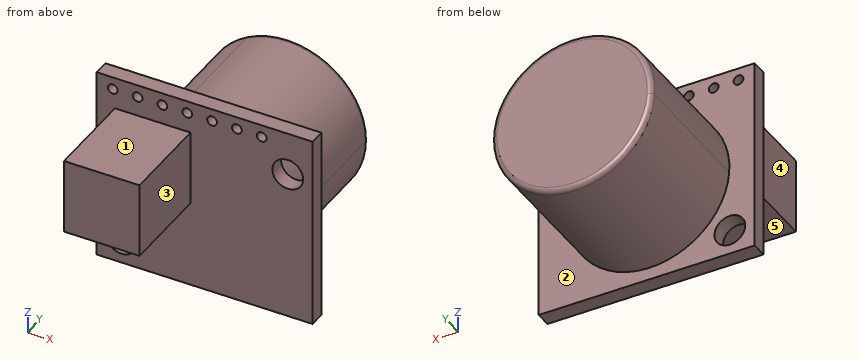
```python
from build123d import *

# Parameters (mm, degrees)
SKETCH1_W           = 22.098
SKETCH1_H           = 19.939
SKETCH1_R           = 0.5
SKETCH1_R_2         = 1.5748
BOSS_EXTRUDE1_DEPTH = 1.6002
SKETCH1_3_W         = 7.7216
SKETCH1_3_H         = 7.7216
BOSS_EXTRUDE2_DEPTH = 9.3472
BOSS_EXTRUDE3_DEPTH = 15.7734
FILLET1_R           = 0.5


with BuildPart() as part:
    # Sketch1 → Boss-Extrude1 (new body)
    # profile 1 of 6: a face of its own
    with BuildSketch(Plane(origin=(0, 0, 0), x_dir=(1, 0, 0), z_dir=(0, 1, 0))):
        with Locations((11.049, 9.9695)):
            Rectangle(SKETCH1_W, SKETCH1_H)
        with Locations(Location((1.651, 1.27, 0), (0, 0, 270))):
            Circle(SKETCH1_R, mode=Mode.SUBTRACT)
        with Locations(Location((4.191, 1.27, 0), (0, 0, 270))):
            Circle(SKETCH1_R, mode=Mode.SUBTRACT)
        with Locations(Location((6.731, 1.27, 0), (0, 0, 270))):
            Circle(SKETCH1_R, mode=Mode.SUBTRACT)
        with Locations(Location((9.271, 1.27, 0), (0, 0, 270))):
            Circle(SKETCH1_R, mode=Mode.SUBTRACT)
        with Locations(Location((11.811, 1.27, 0), (0, 0, 270))):
            Circle(SKETCH1_R, mode=Mode.SUBTRACT)
        with Locations(Location((14.351, 1.27, 0), (0, 0, 270))):
            Circle(SKETCH1_R, mode=Mode.SUBTRACT)
        with Locations(Location((16.891, 1.27, 0), (0, 0, 270))):
            Circle(SKETCH1_R, mode=Mode.SUBTRACT)
        with Locations(Location((19.558, 4.445, 0), (0, 0, 270))):
            Circle(SKETCH1_R_2, mode=Mode.SUBTRACT)
        with BuildLine():
            Line((1.8796, 3.302), (1.8796, 11.0236))
            Line((1.8796, 11.0236), (2.600005352, 11.0236))
            ThreePointArc((2.600005352, 11.0236), (11.040962011, 18.677352606), (18.965620393, 10.4902))
            ThreePointArc((18.965620393, 10.4902), (14.952824562, 3.444697625), (6.845958862, 3.302))
            Line((6.845958862, 3.302), (1.8796, 3.302))
        make_face(mode=Mode.SUBTRACT)
        with Locations(Location((2.54, 17.399, 0), (0, 0, 270))):
            Circle(SKETCH1_R_2, mode=Mode.SUBTRACT)
    # profile 2 of 6: a face of its own
    with BuildSketch(Plane(origin=(0, 0, 0), x_dir=(1, 0, 0), z_dir=(0, 1, 0))):
        with BuildLine():
            Line((2.600005352, 11.0236), (1.8796, 11.0236))
            Line((1.8796, 11.0236), (1.8796, 3.302))
            Line((1.8796, 3.302), (6.845958862, 3.302))
            ThreePointArc((6.845958862, 3.302), (3.596234131, 6.543223808), (2.600005352, 11.0236))
        make_face()
    # profile 3 of 6: a face of its own
    with BuildSketch(Plane(origin=(0, 0, 0), x_dir=(1, 0, 0), z_dir=(0, 1, 0))):
        with BuildLine():
            ThreePointArc((18.965620393, 10.4902), (11.040962011, 18.677352606), (2.600005352, 11.0236))
            Line((2.600005352, 11.0236), (9.6012, 11.0236))
            Line((9.6012, 11.0236), (9.6012, 3.302))
            Line((9.6012, 3.302), (6.845958862, 3.302))
            ThreePointArc((6.845958862, 3.302), (14.952824562, 3.444697625), (18.965620393, 10.4902))
        make_face()
    # profile 4 of 6: a face of its own
    with BuildSketch(Plane(origin=(0, 0, 0), x_dir=(1, 0, 0), z_dir=(0, 1, 0))):
        with BuildLine():
            Line((9.6012, 11.0236), (2.600005352, 11.0236))
            ThreePointArc((2.600005352, 11.0236), (3.596234131, 6.543223808), (6.845958862, 3.302))
            Line((6.845958862, 3.302), (9.6012, 3.302))
            Line((9.6012, 3.302), (9.6012, 11.0236))
        make_face()
    # profile 5 of 6: a face of its own
    with BuildSketch(Plane(origin=(0, 0, 0), x_dir=(1, 0, 0), z_dir=(0, 1, 0))):
        with BuildLine():
            ThreePointArc((18.965620393, 10.4902), (11.040962011, 18.677352606), (2.600005352, 11.0236))
            Line((2.600005352, 11.0236), (9.6012, 11.0236))
            Line((9.6012, 11.0236), (9.6012, 3.302))
            Line((9.6012, 3.302), (6.845958862, 3.302))
            ThreePointArc((6.845958862, 3.302), (14.952824562, 3.444697625), (18.965620393, 10.4902))
        make_face()
    # profile 6 of 6: a face of its own
    with BuildSketch(Plane(origin=(0, 0, 0), x_dir=(1, 0, 0), z_dir=(0, 1, 0))):
        with BuildLine():
            Line((9.6012, 11.0236), (2.600005352, 11.0236))
            ThreePointArc((2.600005352, 11.0236), (3.596234131, 6.543223808), (6.845958862, 3.302))
            Line((6.845958862, 3.302), (9.6012, 3.302))
            Line((9.6012, 3.302), (9.6012, 11.0236))
        make_face()
    extrude(amount=BOSS_EXTRUDE1_DEPTH)

    # Sketch1_3 → Boss-Extrude2 (add)
    with BuildSketch(Plane(origin=(0, 0, 0), x_dir=(1, 0, 0), z_dir=(0, 1, 0))):
        with Locations((5.7404, 7.1628)):
            Rectangle(SKETCH1_3_W, SKETCH1_3_H)
    extrude(amount=-BOSS_EXTRUDE2_DEPTH)

    # Sketch1_4 → Boss-Extrude3 (add)
    with BuildSketch(Plane(origin=(0, 0, 0), x_dir=(1, 0, 0), z_dir=(0, 1, 0))):
        with BuildLine():
            ThreePointArc((18.965620393, 10.4902), (11.040962011, 18.677352606), (2.600005352, 11.0236))
            Line((2.600005352, 11.0236), (9.6012, 11.0236))
            Line((9.6012, 11.0236), (9.6012, 3.302))
            Line((9.6012, 3.302), (6.845958862, 3.302))
            ThreePointArc((6.845958862, 3.302), (14.952824562, 3.444697625), (18.965620393, 10.4902))
        make_face()
        with BuildLine():
            Line((9.6012, 11.0236), (2.600005352, 11.0236))
            ThreePointArc((2.600005352, 11.0236), (3.596234131, 6.543223808), (6.845958862, 3.302))
            Line((6.845958862, 3.302), (9.6012, 3.302))
            Line((9.6012, 3.302), (9.6012, 11.0236))
        make_face()
    extrude(amount=BOSS_EXTRUDE3_DEPTH)

    # Fillet1
    fillet1_edges = [part.edges().sort_by_distance(p)[0] for p in [
        (18.948235433, 15.7734, -9.9568),
    ]]
    fillet(fillet1_edges, radius=FILLET1_R)


solid = part.part
```
For this review, take the finished solid that the model builds, in its own axes (mm). Face numbers are marked on the shaded views. A direction names the side the tool comes from. Coordinates: 2 decimals unless noted, no trailing zeros. Order: outer loops, then holes, each group sorted by start corner. A loop starts at its lowest first (then second) coordinate and runs counter-clockwise, first axis right, second up. Notation, with made-up numbers: (42.5, 48) - (92.5, 48) arc R23 cw to (92.5, 60) - close; hole circle Ø2 at (-17.5, -14.75). An arc over 180 degrees is marked (long way). Answer as a JSON object with one key per item and string values. Group by question number.
1. We need section B-B on y = 12. State the section outline as (x, z) points, then the cut area to 3 significant figures.
2. Clearance check with flat-ended pins moving along their axes: P1, Ø8, axis at x = 13, y = 10, coming from the +Z side; P2, Ø6, axis at x = 7, y = -5.5, coming from the -Z side; P3, Ø2.5, axis at x = 5, y = -5.5, coming from the +Z side. State where each tip first meets the part, or that it passes through.
3. For probe 1 along Y at (x, z) = (17, -13.5); probe 2 along Y at (x, z) = (18, -5); probe 3 along Z at (x, y) = (9.5, -7.75), list the stretches that pass through material, from the lowest coordinate up.
4. We need section A-A on z = -1.27. Give the number of separate pieces and of enclosed holes in the cut face, then the cut area to 3 significant figures.
5. For the marked faces 1, 2, 3, 4 and 5, list the 3-axis set-ups (+Z, -Z, +X, -X, +Y, -Y) from which the entire face can be reached by the end or side of a thin tool; tool diameter is ignored.
Final values:
{
 "1": {"outline": "circle Ø16.38 at (10.77, -10.49)", "area": "211 mm²"},
 "2": {"P1": "z = -2.3", "P2": "z = -11.02", "P3": "z = -3.3"},
 "3": {"probe 1": "0 to 15.77", "probe 2": "0 to 1.6", "probe 3": "-11.02 to -3.3"},
 "4": {"separate pieces": "8", "enclosed holes": "0", "area": "24.2 mm²"},
 "5": {"face 1": "+Z, +X, -X, -Y", "face 2": "+Y", "face 3": "+Z, -Z, +X, -Y", "face 4": "+Z, -Z, -X, -Y", "face 5": "-Z, +X, -X, -Y"}
}
